Design review of the part built by this model. Coordinates are the model's own, in mm. Coordinates: 2 decimals unless noted, no trailing zeros. Write each loop counter-clockwise with the first axis right and the second up, starting at its lowest first coordinate (ties: lowest second). Pieces come first, ordered by that corner, then holes. Notation, with made-up numbers: (63, 31) -> (77, 31) arc R13 cw to (77, 46) -> close; hole circle Ø6 at (-19.75, 31.5). An arc over 180 degrees is marked (long way). Write item = value, one per line. Start each with the question number.
```python
from build123d import *

# Parameters (mm, degrees)
F0_W     = 152.4
F0_H     = 228.6
F0_W_2   = 3
F0_H_2   = 6
F1_DEPTH = 3


with BuildPart() as f1:
    # F0 (on Front) → F1 (new body)
    with BuildSketch(Plane.XZ):
        Polygon((101.6, -133.35), (101.6, 133.35), (50.8, 133.35), (47.8, 133.35), (45.8, 133.35), (42.8, 133.35), (40.8, 133.35), (37.8, 133.35), (-37.8, 133.35), (-37.8, 136.35), (-35.8, 136.35), (-37.8, 139.35), (-40.8, 139.35), (-40.8, 133.35), (-42.8, 133.35), (-42.8, 139.35), (-45.8, 139.35), (-45.8, 133.35), (-47.8, 133.35), (-47.8, 139.35), (-50.8, 139.35), (-52.8, 136.35), (-50.8, 136.35), (-50.8, 133.35), (-101.6, 133.35), (-101.6, -133.35), (-50.8, -133.35), (-50.8, -136.35), (-52.8, -136.35), (-50.8, -139.35), (-47.8, -139.35), (-47.8, -133.35), (-45.8, -133.35), (-45.8, -139.35), (-42.8, -139.35), (-42.8, -133.35), (-40.8, -133.35), (-40.8, -139.35), (-37.8, -139.35), (-35.8, -136.35), (-37.8, -136.35), (-37.8, -133.35), (37.8, -133.35), (37.8, -136.35), (35.8, -136.35), (37.8, -139.35), (40.8, -139.35), (40.8, -133.35), (42.8, -133.35), (42.8, -139.35), (45.8, -139.35), (45.8, -133.35), (47.8, -133.35), (47.8, -139.35), (50.8, -139.35), (52.8, -136.35), (50.8, -136.35), (50.8, -133.35), align=None)
        Rectangle(F0_W, F0_H, mode=Mode.SUBTRACT)
        Polygon((47.8, 133.35), (50.8, 133.35), (50.8, 136.35), (52.8, 136.35), (50.8, 139.35), (47.8, 139.35), align=None)
        with Locations((44.3, 136.35)):
            Rectangle(F0_W_2, F0_H_2)
        Polygon((37.8, 133.35), (40.8, 133.35), (40.8, 139.35), (37.802805, 139.3444), (35.8, 136.3444), (37.8, 136.35), align=None)
    extrude(amount=F1_DEPTH)


solid = f1.part
```
(1) Take a section at B-B, the plane z = 67. State the section outline as (x, y) points, then the cut area to 3 significant figures.
(2) For line 1 (Z direction, x = 8, y = -2.3); line 2 (X direction, y = -0.65, z = 24); line 3 (Z direction, x = 45.5, y = -2.2), list the stretches that pass through material, from the lowest coordinate up.
(3) For pin 1 Ø1.5 at (y, z) = (-1, -137.5) entering from +X; pin 2 Ø0.9 at (y, z) = (-1.5, -136.5) entering from +X; pin 3 Ø1 at (x, y) = (-51.5, -1) entering from -Z, all flat-tipped, find the tip position at first contact; note any pin that passes through.
(4) Take a section at A-A, the plane x = 62.5. State the section outline as (y, z) points.
(5) Take a section at C-C, the plane x = 89.5. State the section outline as (y, z) points, then the cut area to 3 significant figures.
Report:
q1.outline = (-101.6, -3) -> (-76.2, -3) -> (-76.2, 0) -> (-101.6, 0) -> close; (76.2, -3) -> (101.6, -3) -> (101.6, 0) -> (76.2, 0) -> close
q1.area = 152 mm2
q2.line_1 = -133.35 to -114.3, 114.3 to 133.35
q2.line_2 = -101.6 to -76.2, 76.2 to 101.6
q2.line_3 = -139.35 to -114.3, 114.3 to 139.35
q3.pin_1 = 52.53
q3.pin_2 = 52.8
q3.pin_3 = -139.05
q4.outline = (-3, -133.35) -> (0, -133.35) -> (0, -114.3) -> (-3, -114.3) -> close; (-3, 114.3) -> (0, 114.3) -> (0, 133.35) -> (-3, 133.35) -> close
q5.outline = (-3, -133.35) -> (0, -133.35) -> (0, 133.35) -> (-3, 133.35) -> close
q5.area = 800 mm2
